Check sheet for the modelled part. Datum: model origin and axes. Units: mm. A direction names the side the tool comes from. Give positions to 0.01 mm unless a question says otherwise; leave off trailing zeros. Order: outer loops, then holes, each group sorted by start corner. A loop starts at its lowest first (then second) coordinate and runs counter-clockwise, first axis right, second up.
Item 1: Sectioned sample at B-B on x = 0.65. Count the separate pieces of the cut face and the enclosed holes in it, and give its area (3 significant figures).
Item 2: Release check for a two-part mould opening along Y. For faces 5 (the flat face through (2, -11.325, 46)), 6 (the flat face through (2, 15.5, 0)), 7 (the flat face through (2, 12, -47.675)), 8 (the cylindrical face through (1.565, -17.645, 40.577)) record: released by +Y, released by -Y, zero draft, split by the parting line, or undercut.
Item 3: Sectioned sample at A-A on y = 14. Record the boundary of the cut face in (x, z) (3 decimals), and give its area (3 significant figures).
Item 4: Sectioned sample at C-C on z = -16. Record the boundary of the cut face in (x, y) (3 decimals), and give its area (3 significant figures).
Item 5: Material ranges on line 1 along Z through (x, y) = (2.9, -8) (3 decimals); line 2 along Y through (x, z) = (2.95, 38); line 3 along Y through (x, z) = (1.25, 0.5), recorded low to high.
Item 6: Access from +Z, -Z, +X, -X, +Y, -Y to the whole of each face (thin tool, end or side, straight path). Record for faces 1 (the flat face through (2, -14.5, 1)), 2 (the flat face through (2, 15.5, -46)), 3 (the flat face through (0, 0, 1)), 4 (the flat face through (2, 17, -4.825)).
from build123d import *

# Parameters (mm, degrees)
SKETCH1_W           = 99.35
SKETCH1_H           = 37
BOSS_EXTRUDE1_DEPTH = 3.175
SKETCH2_W           = 2.8
SKETCH2_H           = 6
SKETCH2_H_2         = 8
CUT_EXTRUDE1_DEPTH  = 54.103071945
SKETCH3_W           = 79.35
SKETCH3_H           = 4
CUT_EXTRUDE2_DEPTH  = 54.103071945
FILLET1_R           = 3
FILLET2_R           = 0.5
SKETCH4_W           = 9.65
SKETCH4_H           = 3
CUT_EXTRUDE3_DEPTH  = 54.103071945
FILLET3_R           = 0.5


with BuildPart() as part:
    # Sketch1 → Boss-Extrude1 (new body)
    with BuildSketch(Plane(origin=(0, 0, 0), x_dir=(0, 0, -1), z_dir=(1, 0, 0))):
        Rectangle(SKETCH1_W, SKETCH1_H)
    extrude(amount=BOSS_EXTRUDE1_DEPTH)

    # Sketch2 → Cut-Extrude1 (cut, through all)
    with BuildSketch(Plane(origin=(3.175, 0, 0), x_dir=(0, 0, -1), z_dir=(1, 0, 0))):
        with Locations((-46.275, 12.5)):
            Rectangle(SKETCH2_W, SKETCH2_H)
        with Locations((46.275, 12.5)):
            Rectangle(SKETCH2_W, SKETCH2_H)
        with Locations((-46.275, -7.325)):
            Rectangle(SKETCH2_W, SKETCH2_H_2)
        with Locations((46.275, -7.325)):
            Rectangle(SKETCH2_W, SKETCH2_H_2)
    extrude(amount=-CUT_EXTRUDE1_DEPTH, mode=Mode.SUBTRACT)

    # Sketch3 → Cut-Extrude2 (cut, through all)
    with BuildSketch(Plane(origin=(3.175, 0, 0), x_dir=(0, 0, -1), z_dir=(1, 0, 0))):
        with Locations((0, -16.5)):
            Rectangle(SKETCH3_W, SKETCH3_H)
    extrude(amount=-CUT_EXTRUDE2_DEPTH, mode=Mode.SUBTRACT)

    # Fillet1
    fillet1_edges = [part.edges().sort_by_distance(p)[0] for p in [
        (1.5875, -18.5, -49.675),
        (1.5875, -18.5, 49.675),
        (1.5875, -18.5, 39.675),
        (1.5875, -18.5, -39.675),
    ]]
    fillet(fillet1_edges, radius=FILLET1_R)

    # Fillet2
    fillet2_edges = [part.edges().sort_by_distance(p)[0] for p in [
        (1.5875, 18.5, 49.675),
        (1.5875, 18.5, -49.675),
        (1.5875, -14.5, 39.675),
        (1.5875, -14.5, -39.675),
    ]]
    fillet(fillet2_edges, radius=FILLET2_R)

    # Sketch4 → Cut-Extrude3 (cut, through all)
    with BuildSketch(Plane(origin=(3.175, 0, 0), x_dir=(0, 0, -1), z_dir=(1, 0, 0))):
        with Locations((0, 17)):
            Rectangle(SKETCH4_W, SKETCH4_H)
    extrude(amount=-CUT_EXTRUDE3_DEPTH, mode=Mode.SUBTRACT)

    # Fillet3
    fillet3_edges = [part.edges().sort_by_distance(p)[0] for p in [
        (1.5875, 18.5, 4.825),
        (1.5875, 18.5, -4.825),
    ]]
    fillet(fillet3_edges, radius=FILLET3_R)


solid = part.part
Report:
1. separate pieces: 1
1. enclosed holes: 4
1. area: 3,240 mm2
2. face 5: undercut
2. face 6: released by +Y
2. face 7: undercut
2. face 8: released by -Y
3. outline: (0, -49.675) - (3.175, -49.675) - (3.175, -47.675) - (0, -47.675) - close; (0, -44.875) - (3.175, -44.875) - (3.175, 44.875) - (0, 44.875) - close; (0, 47.675) - (3.175, 47.675) - (3.175, 49.675) - (0, 49.675) - close
3. area: 298 mm2
4. outline: (0, -14.5) - (3.175, -14.5) - (3.175, 18.5) - (0, 18.5) - close
4. area: 105 mm2
5. line 1: z = -49.675 to -47.675, -44.875 to 44.875, 47.675 to 49.675
5. line 2: y = -14.5 to 18.5
5. line 3: y = -14.5 to 15.5
6. face 1: +X, -X, -Y
6. face 2: +X, -X
6. face 3: +Z, -Z, -X, +Y, -Y
6. face 4: +X, -X, +Y
